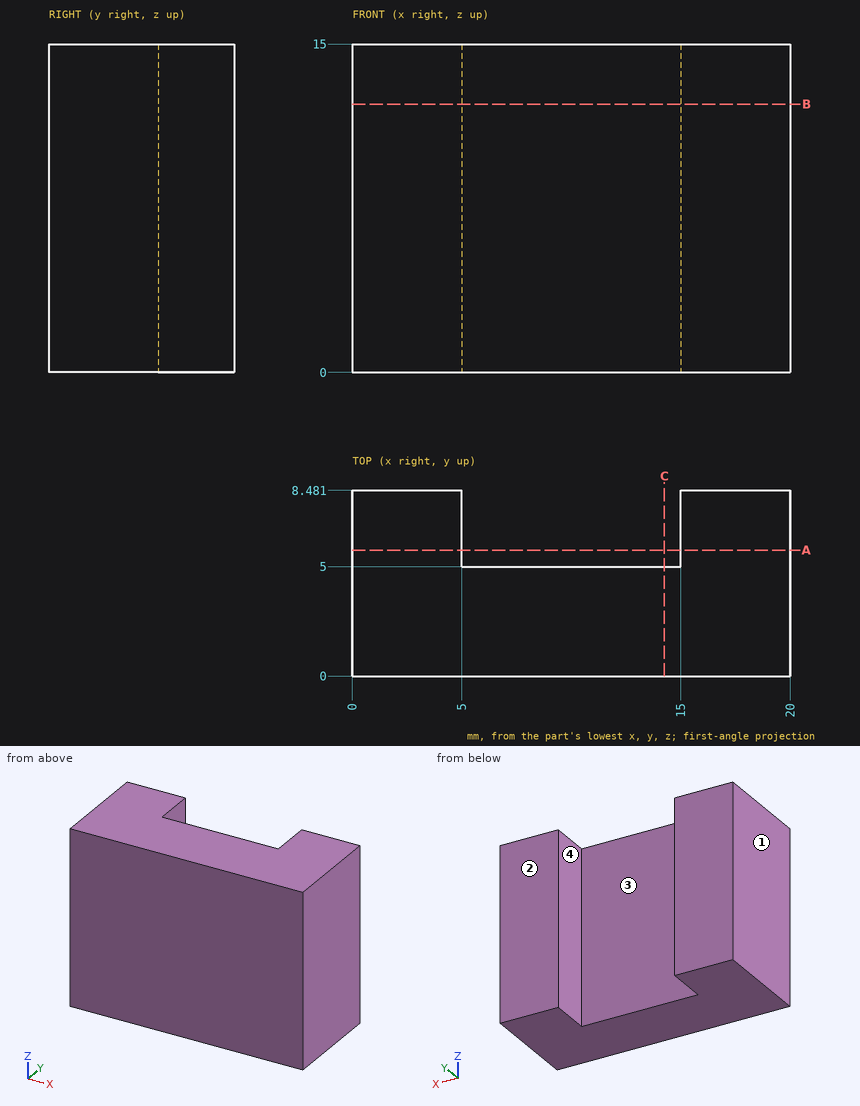
Geometry check sheet. Reference: drawing and pictorial views, mm from the part's lowest x, y, z. Coordinates: 2 decimals unless noted, no trailing zeros. Loops run counter-clockwise (first coordinate to the right, second up) from the corner with the lowest first, then second, coordinate; pieces in that order, holes last. Notation, with made-up numbers: (84.25, -38.5) - (137.25, -38.5) arc R27 cw to (137.25, -4.5) - close; hole circle Ø10 at (-15, -5). An arc over 180 degrees is marked (long way). Return JSON: item names as keys, results as strings.
1. Go/stop test with a flat-tipped pin: pin 1 (5 mm diameter, centred on x = 11.5, z = 8.5, fed in from +Y). Record where the tip stops, or that it passes through.
Established:
{"pin 1": "stops at y = 5"}
2. Mould release check, pull along X, two halves, no side actions. Record for the marked faces 1, 2, 3 and 4: +X half, -X half, draft (parallel to the pull), parting line (faces both ways), or undercut.
Established:
{"face 1": "-X half", "face 2": "draft", "face 3": "undercut", "face 4": "undercut"}
3. Thickness scan on L1, parallel to X at y = 6.25, z = 1; L2, parallel to Y at x = 11.5, z = 7.25. Record the ranges inside material, lowest first.
Established:
{"L1": "x = 0 to 5, 15 to 20", "L2": "y = 0 to 5"}
4. Section check B-B, the plane z = 12.25. Record the boundary of the cut face in (x, y), then the cut area to 3 significant figures.
Established:
{"outline": "(0, 0) - (20, 0) - (20, 8.48) - (15, 8.48) - (15, 5) - (5, 5) - (5, 8.48) - (0, 8.48) - close", "area": "135 mm2"}
5. Section check A-A, the plane y = 5.75. Record the boundary of the cut face in (x, z).
Established:
{"outline": "(0, 0) - (5, 0) - (5, 15) - (0, 15) - close; (15, 0) - (20, 0) - (20, 15) - (15, 15) - close"}
6. Section check C-C, the plane x = 14.25. Record the boundary of the cut face in (y, z).
Established:
{"outline": "(0, 0) - (5, 0) - (5, 15) - (0, 15) - close"}
